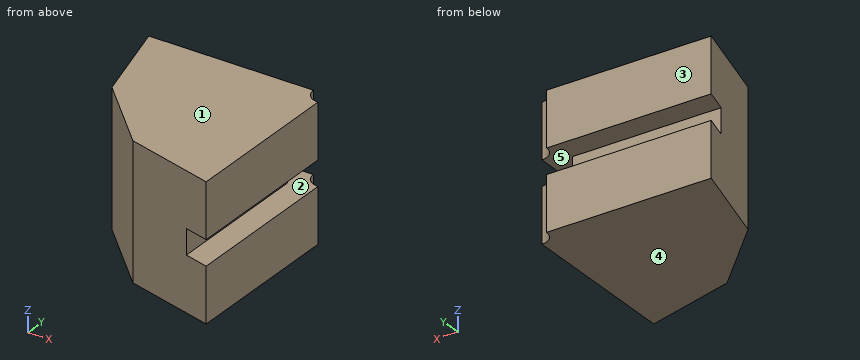
```python
from build123d import *

# Parameters (mm, degrees)
F1_DEPTH = 38.1
F3_W     = 50.8
F3_H     = 7.112
F4_DEPTH = 6.858
F2_W     = 50.8
F2_H     = 7.112
F5_DEPTH = 6.858
F6_R     = 4.1275
F7_DEPTH = 39.624


with BuildPart() as f1:
    # F0 (on Top) → F1 (new body)
    with BuildSketch(Plane.XY):
        Polygon((-25.4, -43.994091), (0, -50.8), (0, 0), (-50.8, 0), (-43.994091, -25.4), align=None)
    extrude(amount=F1_DEPTH)

    # F3 (on face) → F4 (cut)
    with BuildSketch(Plane.YZ):
        with Locations((-25.4, 19.05)):
            Rectangle(F3_W, F3_H)
    extrude(amount=-F4_DEPTH, mode=Mode.SUBTRACT)

    # F2 (on face) → F5 (cut)
    with BuildSketch(Plane(origin=(0, 0, 0), x_dir=(-1, 0, 0), z_dir=(0, 1, 0))):
        with Locations((25.4, 19.05)):
            Rectangle(F2_W, F2_H)
    extrude(amount=-F5_DEPTH, mode=Mode.SUBTRACT)

    # F6 (on face) → F7 (cut)
    with BuildSketch(Plane.XY.offset(38.1)):
        Circle(F6_R)
    extrude(amount=-F7_DEPTH, mode=Mode.SUBTRACT)


solid = f1.part
```
Input: part model. Units: mm. Frame: model coordinates. Face numbers are marked on the shaded views. A direction names the side the tool comes from. Coordinates: 2 decimals unless noted, no trailing zeros. Write each loop counter-clockwise with the first axis right and the second up, starting at its lowest first coordinate (ties: lowest second). Pieces come first, ordered by that corner, then holes. Notation, with made-up numbers: (-6.75, 22) -> (1.25, 22) arc R21 cw to (1.25, 58) -> close; hole circle Ø9 at (6, 7). An arc over 180 degrees is marked (long way). Answer as a JSON object with one key per item and string values.
1. First-contact query: P1, Ø3, axis at x = -41, z = 29.5, coming from the -Y side; P2, Ø3.5, axis at y = -35.5, z = 18.5, coming from the +X side; P3, Ø3, axis at y = -15.5, z = 24, coming from the -X side. Flat tips, straight axial feed; report the tip coordinate or a pass-through.
Result set:
{"P1": "stops at y = -29.89", "P2": "stops at x = -6.86", "P3": "stops at x = -47.05"}
2. Section A-A on z = 18. Return the cut outline in (x, y).
Result set:
{"outline": "(-48.96, -6.86) -> (-43.99, -25.4) -> (-25.4, -43.99) -> (-6.86, -48.96) -> (-6.86, -6.86) -> close"}
3. Section D-D on z = 7. Return the cut outline in (x, y) (1 decimal), then the cut area to 3 significant figures.
Result set:
{"outline": "(-50.8, 0) -> (-44, -25.4) -> (-25.4, -44) -> (0, -50.8) -> (0, -4.1) arc R4.1 cw to (-4.1, 0) -> close", "area": "1,920 mm2"}
4. Access query for the marked faces 1 and 2. Directions: +Z, -Z, +X, -X, +Y, -Y. A direction counts if a zero-diameter tool reaches every point of the face in a straight line with its end or side. Return the directions, or none.
Result set:
{"face 1": "+Z, +X, -X, +Y, -Y", "face 2": "+X, +Y"}
5. Section C-C on y = -17.5. Return the cut outline in (x, z).
Result set:
{"outline": "(-46.11, 0) -> (0, 0) -> (0, 15.49) -> (-6.86, 15.49) -> (-6.86, 22.61) -> (0, 22.61) -> (0, 38.1) -> (-46.11, 38.1) -> close"}
6. Material intervals for line 1 (Z direction, x = -40.5, y = -2.5); line 2 (X direction, y = -10, z = 22); line 3 (X direction, y = -27, z = 13.5), sorted ascending. Write a range as from..to.
Result set:
{"line 1": "z = 0..15.49, 22.61..38.1", "line 2": "x = -48.12..-6.86", "line 3": "x = -42.39..0"}
7. Section B-B on x = -17. Return the cut outline in (y, z), then the cut area to 3 significant figures.
Result set:
{"outline": "(-46.24, 0) -> (0, 0) -> (0, 15.49) -> (-6.86, 15.49) -> (-6.86, 22.61) -> (0, 22.61) -> (0, 38.1) -> (-46.24, 38.1) -> close", "area": "1,710 mm2"}
8. Mould query, pull axis Z, two halves, no side actions, for the marked faces 3, 4 and 5. Classes: released by +Z, released by -Z, zero draft, split by the parting line, or undercut.
Result set:
{"face 3": "zero draft", "face 4": "released by -Z", "face 5": "undercut"}
